Can you work these out from the model? Positions are in its coordinate system, mm. Face numbers are marked on the shaded views. A direction names the side the tool comes from. Round coordinates to 2 decimals unless told otherwise and drop trailing zeros. Order: outer loops, then holes, each group sorted by start corner. A loop starts at its lowest first (then second) coordinate and runs counter-clockwise, first axis right, second up. Notation, with made-up numbers: (77, -18.5) - (115, -18.5) arc R7 cw to (115, -6.5) - close; hole circle Ø7 at (73, 66.25). An arc over 180 degrees is marked (long way). Write item = value, one per line.
Autodesk Inventor part; units mm, degrees
ref_plane "YZ Plane" through (0, 0, 0) normal (1, 0, 0) x (0, 1, 0)
ref_plane "XZ Plane" through (0, 0, 0) normal (0, 1, 0) x (-1, 0, 0)
ref_plane "XY Plane" through (0, 0, 0) normal (0, 0, 1) x (1, 0, 0)
sketch "Boceto1" plane through (0, 0, 0) normal (0, 1, 0) x (-1, 0, 0)
  circle A0 centre (0, 0) radius 3.15
  circle A1 centre (0, 0) radius 15
  line L0 (-7.225, 3.7) -> (-10.925, 3.7)
  line L1 (-10.925, 3.7) -> (-10.925, -3.7)
  line L2 (-10.925, -3.7) -> (-7.225, -3.7)
  line L3 (-7.225, -3.7) -> (-7.225, 3.7)
  circle A2 centre (0, 0) radius 9.8003 construction
  line L4 (6.8168, -4.407) -> (0.4082, -8.107)
  line L5 (8.6668, -7.6113) -> (6.8168, -4.407)
  line L6 (2.2582, -11.3113) -> (8.6668, -7.6113)
  line L7 (0.4082, -8.107) -> (2.2582, -11.3113)
  line L8 (0.4082, 8.107) -> (6.8168, 4.407)
  line L9 (2.2582, 11.3113) -> (0.4082, 8.107)
  line L10 (8.6668, 7.6113) -> (2.2582, 11.3113)
  line L11 (6.8168, 4.407) -> (8.6668, 7.6113)
  point P0 (-7.225, 0)
  point P1 (-9.075, 3.7)
  point P2 (3.6125, -6.257)
  point P3 (1.3332, -9.7092)
  point P4 (3.6125, 6.257)
  point P5 (7.7418, 6.0092)
  dimension "d0" = 6.3
  dimension "tuerca" = 7.4
  dimension "d2" = 11.85
  dimension "d3" = 6.6503
  dimension "d4" = 3.7
  dimension "d18" = 360
  dimension "d26" = 30
  dimension "d27" = 4.075
  dimension "d28" = 4.075
extrude "Extrusión1" add sketch "Boceto1" along normal blind 10 contours A1 | L5 L6 L7 L4 | L9 L10 L11 L8
sketch "Boceto2" plane through (7.225, 0, -3.7) normal (1, 0, 0) x (0, 0, -1)
  line L0 (0, 0) -> (-7.4, 0)
  line L1 (0, 0) -> (0, 10) construction
  line L2 (-7.4, 10) -> (0, 10) construction
  line L3 (-7.4, 0) -> (-7.4, 10) construction
  line L4 (-7.4, 0) -> (0, 10) construction
  circle A0 centre (-3.7, 5) radius 2.1
  line L5 (0, 2.6329) -> (-4.5603, 0)
  line L6 (-2.8397, 0) -> (-7.4, 2.6329)
  line L7 (-7.4, 2.6329) -> (-7.4, 0)
  line L8 (0, 2.6329) -> (0, 0)
  point P0 (-3.7, 0)
  dimension "d7" = 4.2
  dimension "d8" = 120
  dimension "d9" = 3.9
extrude "Extrusión2" cut sketch "Boceto2" along normal mid plane 16 contours A0
extrude "Extrusión3" add sketch "Boceto2" along normal up to next contours L0 L6 L5 L8 | L0 L5 L6 | L0 L7 L6 L5
sketch "Boceto3" plane through (0, 0, 0) normal (0, -1, 0) x (1, 0, 0)
  circle A0 centre (0, 0) radius 3.15
  circle A1 centre (0, 0) radius 27.5
  line L0 (-8, 8) -> (8, 8)
  line L1 (8, 8) -> (8, -8)
  line L2 (8, -8) -> (-8, -8)
  line L3 (-8, -8) -> (-8, 8)
  point P0 (-8, 0)
  point P1 (0, 8)
  dimension "d32" = 16
  dimension "d33" = 55
extrude "Extrusión4" add sketch "Boceto3" along normal blind 8 contours L0 L1 L2 L3
chamfer "Chaflán1" distance 1 angle 45 2 edges at (9.075, 10, 3.7) (9.075, 10, -3.7)
chamfer "Chaflán3" distance 1 angle 45 4 edges at (0, -8, 8) (-8, -8, 0) (0, -8, -8) (8, -8, 0)
equation "\"d28\" = d27"
properties part number "dado polea"
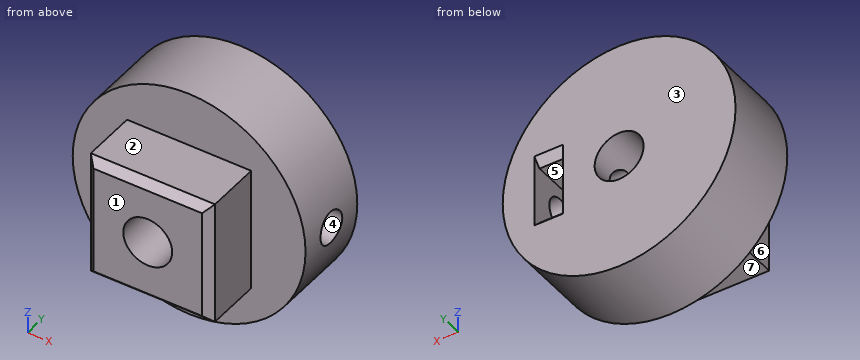
(1) Thinking about a two-plate mould opening in Y: for the marked faces 1, 2, 3 and 4, which applies, +Y half, -Y half, draft (parallel to the pull), parting line (faces both ways), or undercut?
Computed:
face_1 = -Y half
face_2 = draft
face_3 = +Y half
face_4 = undercut
(2) If we section it at C-C (y = 4): Write out the boundary of the cut face in (x, z) (3 decimals), plus the area to 3 significant figures.
Computed:
outline = (2.552, -1.847) arc R3.15 cw (long way) to (2.552, 1.847) - (7.225, 1.847) - (7.225, 3.7) - (10.925, 3.7) - (10.925, 1.847) - (14.886, 1.847) arc R15 ccw (long way) to (14.886, -1.847) - (10.925, -1.847) - (10.925, -3.7) - (7.225, -3.7) - (7.225, -1.847) - close
area = 618 mm^2
(3) If I drill on line 1 (X direction, y = 7.75, z = 0) (3 decimals); line 2 (Y direction, x = 13, z = 0); line 3 (Y direction, x = 5, z = 0), over which ranges is the centre line in solid material (lowest first)? Write a range as from..to.
Computed:
line_1 = -15..-3.15, 3.15..7.225, 10.925..15
line_2 = 0..2.9, 7.1..10
line_3 = -8..2.9, 7.1..10
(4) On a 3-axis mill with a long thin cutter (end or side, diameter ignored), from which of +Z, -Z, +X, -X, +Y, -Y can I reach the whole of each face in a straight line? I mean the marked faces 5, 6 and 7. Say none if no direction works.
Computed:
face_5 = +Y
face_6 = +Z, -Z, -X, -Y
face_7 = -Z, +X, -X, -Y
(5) If we section it at B-B (y = -0.75): Write out the boundary of the cut face in (x, z).
Computed:
outline = (-8, -8) - (8, -8) - (8, 8) - (-8, 8) - close; hole circle Ø6.3 at (0, 0)
(6) If we section it at A-A (x = 0): Write out the boundary of the cut face in (y, z), plus the area to 3 significant figures.
Computed:
outline = (-8, -7) - (-7, -8) - (0, -8) - (0, -15) - (10, -15) - (10, -3.15) - (-8, -3.15) - close; (-8, 3.15) - (10, 3.15) - (10, 15) - (0, 15) - (0, 8) - (-7, 8) - (-8, 7) - close
area = 314 mm^2
(7) If we section it at D-D (x = -6): Write out the boundary of the cut face in (y, z), plus the area to 3 significant figures.
Computed:
outline = (-8, -7) - (-7, -8) - (0, -8) - (0, -13.75) - (10, -13.75) - (10, 13.75) - (0, 13.75) - (0, 8) - (-7, 8) - (-8, 7) - close
area = 402 mm^2
(8) Will these pins go through, and if not, where does the flat tip stop? P1, Ø3.5, axis at y = 5, z = 0, coming from the +X side; P2, Ø3, axis at x = 8.5, y = 6.5, coming from the -Z side; P3, Ø3.5, axis at x = -3, y = -4.5, coming from the -Z side.
Computed:
P1 = -2.62
P2 = -13.27
P3 = -8
